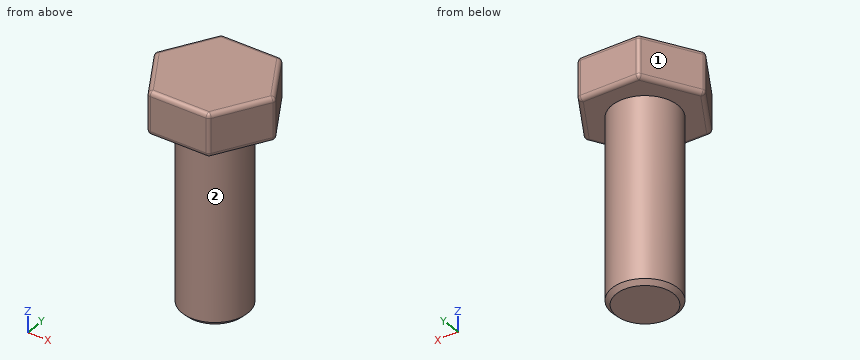
Autodesk Inventor part; units mm, degrees
ref_plane "YZ Plane" through (0, 0, 0) normal (1, 0, 0) x (0, 1, 0)
ref_plane "XZ Plane" through (0, 0, 0) normal (0, 1, 0) x (-1, 0, 0)
ref_plane "XY Plane" through (0, 0, 0) normal (0, 0, 1) x (1, 0, 0)
sketch "Sketch1" plane through (0, 0, 0) normal (0, 0, 1) x (1, 0, 0)
  circle A0 centre (0, 0) radius 3.9688
  dimension "d0" = 7.9375
extrude "Extrusion1" add sketch "Sketch1" against normal blind 22.225
sketch "Sketch2" plane through (0, 0, 0) normal (0, 0, 1) x (1, 0, 0)
  circle A0 centre (0, 0) radius 3.9687
  line L0 (-7.3323, 0) -> (-3.6662, 6.35)
  line L1 (-3.6662, 6.35) -> (3.6662, 6.35)
  line L2 (3.6662, 6.35) -> (7.3323, 0)
  line L3 (7.3323, 0) -> (3.6662, -6.35)
  line L4 (3.6662, -6.35) -> (-3.6662, -6.35)
  line L5 (-3.6662, -6.35) -> (-7.3323, 0)
  dimension "d3" = 12.7
extrude "Extrusion2" add sketch "Sketch2" along normal blind 5.1594 contours A0 | L0 L1 L2 L3 L4 L5
thread "Thread1"
chamfer "Chamfer1" distance 0.508 angle 45 1 edges at (-3.9688, 0, -22.225)
fillet "Fillet1" radius 0.508 18 edges at (0, 6.35, 5.1594) (-5.4993, 3.175, 5.1594) (-5.4993, -3.175, 5.1594) (0, -6.35, 5.1594) (5.4993, -3.175, 5.1594) (5.4993, 3.175, 5.1594) (-5.4993, 3.175, 0) (0, 6.35, 0) (5.4993, 3.175, 0) (5.4993, -3.175, 0) (0, -6.35, 0) (-5.4993, -3.175, 0) (7.3323, 0, 2.5797) (3.6662, -6.35, 2.5797) (3.6662, 6.35, 2.5797) (-3.6662, -6.35, 2.5797) (-7.3323, 0, 2.5797) (-3.6662, 6.35, 2.5797)
properties part number "375 bolt x4" material "Steel"
Model file for the job. Use its own axes, mm. Face numbers are marked on the shaded views. A direction names the side the tool comes from. Round coordinates to 2 decimals unless told otherwise and drop trailing zeros. Write each loop counter-clockwise with the first axis right and the second up, starting at its lowest first coordinate (ties: lowest second). Pieces come first, ordered by that corner, then holes. Notation, with made-up numbers: (28.25, -4.5) - (78.25, -4.5) arc R23 cw to (78.25, 28.5) - close; hole circle Ø3 at (26.5, 67.5). An arc over 180 degrees is marked (long way). Use CSV: the item, a comma, the result in double quotes. Start each with the question number.
Item 1: Pin check, flat tips, straight feed: P1, Ø3, axis at x = 2, z = -17.5, coming from the +Y side; P2, Ø4, axis at y = 3.5, z = -0.5, coming from the -X side; P3, Ø2, axis at y = 3.5, z = 0, coming from the -X side; P4, Ø1, axis at y = 4.5, z = -10.5, coming from the -X side. Stop position of each tip, or through.
Item 2: Tool access for the marked faces 1 and 2: list every direction of +Z, -Z, +X, -X, +Y, -Y with a clear straight run to the whole face (end or side of a thin tool).
Item 3: Band-saw the part on B-B (z = -4.25). Write the cut outline in (x, y), and give its area (3 significant figures).
Item 4: Drill centre lines: L1, parallel to Z at x = 3.75, y = -2.5; L2, parallel to Y at x = 0, z = -20.5; L3, parallel to X at y = 2, z = -16. Where is each one in solid material? Low to high. Write a range as [from, to].
Item 5: Band-saw the part on A-A (x = 0). Write the cut outline in (y, z) (3 decimals).
Checked values:
1,P1,"stops at y = 3.94"
1,P2,"stops at x = -6.33"
1,P3,"stops at x = -5.83"
1,P4,"passes through"
2,face 1,"+Z, -Z, -X, +Y"
2,face 2,"-Z"
3,outline,"circle Ø7.94 at (0, 0)"
3,area,"49.5 mm²"
4,L1,"z = [0, 5.16]"
4,L2,"y = [-3.97, 3.97]"
4,L3,"x = [-3.43, 3.43]"
5,outline,"(-6.35, 0.508) arc R0.508 ccw to (-5.842, 0) - (-3.969, 0) - (-3.969, -21.717) - (-3.461, -22.225) - (3.461, -22.225) - (3.969, -21.717) - (3.969, 0) - (5.842, 0) arc R0.508 ccw to (6.35, 0.508) - (6.35, 4.651) arc R0.508 ccw to (5.842, 5.159) - (-5.842, 5.159) arc R0.508 ccw to (-6.35, 4.651) - close"
